Autodesk Inventor part; units mm, degrees
ref_plane "YZ Plane" through (0, 0, 0) normal (1, 0, 0) x (0, 1, 0)
ref_plane "XZ Plane" through (0, 0, 0) normal (0, 1, 0) x (-1, 0, 0)
ref_plane "XY Plane" through (0, 0, 0) normal (0, 0, 1) x (1, 0, 0)
sketch "스케치1" plane through (0, 0, 0) normal (0, 0, 1) x (1, 0, 0)
  circle A0 centre (88.547, 17.9758) radius 1.2
  circle A1 centre (86.2038, 23.6326) radius 1.2
  circle A2 centre (80.547, 25.9758) radius 1.2
  circle A3 centre (74.8901, 23.6326) radius 1.2
  circle A4 centre (72.547, 17.9758) radius 1.2
  circle A5 centre (80.547, 17.9758) radius 5.8
  arc A6 (69.647, 17.9758) -> (74.747, 17.9758) centre (72.197, 18.4832) ccw
  arc A7 (86.347, 17.9758) -> (91.447, 17.9758) centre (88.897, 18.4832) ccw
  line L0 (69.647, 17.9758) -> (91.447, 17.9758)
  line L1 (91.447, 17.9758) -> (91.447, 37.9758)
  line L2 (91.447, 37.9758) -> (69.647, 37.9758)
  line L3 (69.647, 37.9758) -> (69.647, 17.9758)
  line L4 (69.647, 37.9758) -> (99.4042, 37.9758) construction
  line L5 (69.647, 37.9758) -> (91.447, 37.9758)
  line L6 (91.447, 37.9758) -> (91.447, 52.9758)
  line L7 (91.447, 52.9758) -> (69.647, 52.9758)
  line L8 (69.647, 52.9758) -> (69.647, 37.9758)
  line L9 (69.647, 52.9758) -> (69.647, 52.9758)
  line L10 (91.447, 52.9758) -> (91.447, 52.9758)
  circle A8 centre (69.647, 52.9758) radius 21.8
  line L11 (69.647, 52.9758) -> (54.232, 68.3907)
  point P0 (0, 0)
  point P1 (80.547, 17.9758)
  point P2 (80.547, 17.9758)
  point P3 (69.647, 57.9758)
  point P4 (85.4659, 37.9758)
  point P5 (69.647, 31.1758)
  dimension "d4" = 2.6
  dimension "d5" = 2.6
  dimension "d6" = 20
  dimension "d9" = 15
  dimension "d19" = 0
  dimension "d20" = 0
  dimension "d30" = 135
extrude "돌출1" add sketch "스케치1" along normal blind 6 contours L0 A7 A0 | A0 L0 A5 A4 L3 A8 L2 L1 | L2 A8 L6 | A6 L0 A4 | A8 L3 L2 | L2 L8 L7 A8 | L7 L11 A8
sketch "스케치2" plane through (0, 0, 6) normal (0, 0, 1) x (1, 0, 0)
  arc A0 (69.647, 17.9758) -> (74.747, 17.9758) centre (72.197, 18.4832) ccw
  arc A1 (86.347, 17.9758) -> (74.747, 17.9758) centre (80.547, 17.9758) ccw
  arc A2 (86.347, 17.9758) -> (91.447, 17.9758) centre (88.897, 18.4832) ccw
  circle A3 centre (88.547, 17.9758) radius 1.2
  circle A4 centre (72.547, 17.9758) radius 1.2
  circle A5 centre (80.547, 25.9758) radius 1.2
  circle A6 centre (86.2038, 23.6326) radius 1.2
  circle A7 centre (74.8901, 23.6326) radius 1.2
  circle A8 centre (72.547, 17.9758) radius 1.35
  circle A9 centre (74.8901, 23.6326) radius 1.35
  circle A10 centre (80.547, 25.9758) radius 1.35
  circle A11 centre (86.2038, 23.6326) radius 1.35
  circle A12 centre (88.547, 17.9758) radius 1.35
  arc A13 (91.447, 52.9758) -> (54.232, 68.3907) centre (69.647, 52.9758) ccw
  line L0 (69.647, 52.9758) -> (69.647, 17.9758)
  line L1 (91.447, 17.9758) -> (91.447, 52.9758)
  line L2 (54.232, 68.3907) -> (69.647, 52.9758)
  point P0 (0, 0)
  dimension "d12" = 2.7
  dimension "d13" = 2.7
  dimension "d14" = 2.7
  dimension "d15" = 2.7
  dimension "d16" = 2.7
extrude "돌출2" cut sketch "스케치2" against normal blind 6 contours A3 | A4 | A5 | A6 | A7 | A8 | A9 | A10 | A11 | A12
fillet "모깎기1" radius 1 1 edges at (54.232, 68.3907, 3)
sketch "스케치3" plane through (0, 0, 6) normal (0, 0, 1) x (1, 0, 0)
  arc A0 (54.991, 69.114) -> (54.9562, 67.6666) centre (55.6633, 68.3737) ccw
  line L0 (54.9562, 67.6666) -> (69.647, 52.9758)
  line L1 (69.647, 52.9758) -> (69.647, 17.9758)
  arc A1 (69.647, 17.9758) -> (74.747, 17.9758) centre (72.197, 18.4832) ccw
  arc A2 (86.347, 17.9758) -> (74.747, 17.9758) centre (80.547, 17.9758) ccw
  arc A3 (86.347, 17.9758) -> (91.447, 17.9758) centre (88.897, 18.4832) ccw
  line L2 (91.447, 17.9758) -> (91.447, 52.9758)
  arc A4 (91.447, 52.9758) -> (54.991, 69.114) centre (69.647, 52.9758) ccw
  circle A5 centre (86.2038, 23.6326) radius 1.35
  circle A6 centre (88.547, 17.9758) radius 1.35
  circle A7 centre (80.547, 25.9758) radius 1.35
  circle A8 centre (72.547, 17.9758) radius 1.35
  circle A9 centre (74.8901, 23.6326) radius 1.35
  line L3 (85.547, 49.9758) -> (75.547, 49.9758)
  line L4 (75.547, 49.9758) -> (75.547, 55.9758)
  line L5 (75.547, 55.9758) -> (85.547, 55.9758)
  line L6 (85.547, 55.9758) -> (85.547, 49.9758)
  line L7 (85.547, 49.9758) -> (75.547, 55.9758) construction
  line L8 (75.547, 49.9758) -> (85.547, 55.9758) construction
  point P0 (0, 0)
  point P1 (80.547, 52.9758)
  dimension "d22" = 10
  dimension "d23" = 6
extrude "돌출3" cut sketch "스케치3" against normal blind 6 contours L3 L4 L5 L6
sketch "스케치4" plane through (0, 0, 6) normal (0, 0, 1) x (1, 0, 0)
  line L0 (75.547, 49.9758) -> (75.547, 55.9758)
  line L1 (75.547, 55.9758) -> (85.547, 55.9758)
  line L2 (85.547, 55.9758) -> (85.547, 49.9758)
  line L3 (85.547, 49.9758) -> (75.547, 49.9758)
  arc A0 (54.991, 69.114) -> (54.9562, 67.6666) centre (55.6633, 68.3737) ccw
  line L4 (54.9562, 67.6666) -> (69.647, 52.9758)
  line L5 (69.647, 52.9758) -> (69.647, 17.9758)
  arc A1 (69.647, 17.9758) -> (74.747, 17.9758) centre (72.197, 18.4832) ccw
  arc A2 (86.347, 17.9758) -> (74.747, 17.9758) centre (80.547, 17.9758) ccw
  arc A3 (86.347, 17.9758) -> (91.447, 17.9758) centre (88.897, 18.4832) ccw
  line L6 (91.447, 17.9758) -> (91.447, 52.9758)
  arc A4 (91.447, 52.9758) -> (54.991, 69.114) centre (69.647, 52.9758) ccw
  circle A5 centre (86.2038, 23.6326) radius 1.35
  circle A6 centre (88.547, 17.9758) radius 1.35
  circle A7 centre (80.547, 25.9758) radius 1.35
  circle A8 centre (72.547, 17.9758) radius 1.35
  circle A9 centre (74.8901, 23.6326) radius 1.35
  circle A10 centre (72.547, 52.9758) radius 1.35
  circle A11 centre (88.547, 52.9758) radius 1.35
  point P0 (0, 0)
  point P1 (75.547, 52.9758)
  dimension "d26" = 2.7
  dimension "d27" = 2.7
  dimension "d31" = 3
extrude "돌출4" cut sketch "스케치4" against normal blind 6 contours A10 | A11
sketch "스케치5" plane through (0, 0, 6) normal (0, 0, 1) x (1, 0, 0)
  line L0 (75.547, 55.9758) -> (75.547, 49.9758)
  circle A0 centre (75.547, 55.9758) radius 0.75
  circle A1 centre (85.3736, 55.9758) radius 0.75
  line L1 (75.547, 49.9758) -> (85.547, 49.9758)
  circle A2 centre (75.547, 49.9758) radius 0.75
  line L2 (85.547, 49.9758) -> (85.547, 55.9758)
  circle A3 centre (85.547, 49.9758) radius 0.75
  point P0 (0, 0)
  point P1 (85.547, 50.7258)
  point P2 (84.797, 49.9758)
  dimension "d32" = 1.5
  dimension "d33" = 1.5
  dimension "d34" = 1.5
  dimension "d35" = 1.5
extrude "돌출5" cut sketch "스케치5" against normal blind 10 contours A1 | L1 L2 A3 | A2 L1 L0 | L0 L1 A2 | A0 picked at (85.0543, 49.916)
properties part number "frame_hand1" material "PMMA 플라스틱"
Can you work these out from the model? Positions are in its coordinate system, mm. A direction names the side the tool comes from. Round coordinates to 2 decimals unless told otherwise and drop trailing zeros. Write each loop counter-clockwise with the first axis right and the second up, starting at its lowest first coordinate (ties: lowest second). Pieces come first, ordered by that corner, then holes. Notation, with made-up numbers: M -3.75,7 L 53.25,7 A32 cw 53.25,45 Z; hole C 67,-5.75 d9. An arc over 180 degrees is marked long. Use a Markdown table: item, result.
Item 1: For pin 1 Ø1.5 at (x, z) = (59, 3.5) entering from -Y; pin 2 Ø1.5 at (x, z) = (84, 1.5) entering from -Y; pin 3 Ø1 at (y, z) = (55, 3) entering from +X, each with a flat end and sliding along its axis, tell me the tip position at first contact or that it passes through.
Found:
| item | result |
|---|---|
| pin 1 | stops at y = 62.87 |
| pin 2 | stops at y = 21.97 |
| pin 3 | stops at x = 91.39 |
Item 2: Which directions (+Z, -Z, +X, -X, +Y, -Y) give clear straight access to the entire face, cutting with the end or side of a thin tool? Please do faces 4 (the face through (77, 46, 0)), 5 (the face through (80, 55.976, 3)).
Found:
| item | result |
|---|---|
| face 4 | -Z, +X, -X, +Y, -Y |
| face 5 | +Z, -Z |
Item 3: I want a section at D-D (x = 77.5). List the corners of the cut face in (y, z) for me.
Found:
| item | result |
|---|---|
| outline | M 22.91,0 L 49.98,0 L 49.98,6 L 22.91,6 Z; M 55.98,0 L 73.31,0 L 73.31,6 L 55.98,6 Z |
Item 4: I want a section at A-A (x = 83). List the corners of the cut face in (y, z) for me.
Found:
| item | result |
|---|---|
| outline | M 23.23,0 L 49.98,0 L 49.98,6 L 23.23,6 Z; M 55.98,0 L 70.21,0 L 70.21,6 L 55.98,6 Z |
Item 5: I want a section at C-C (y = 32). List the corners of the cut face in (x, z) for me.
Found:
| item | result |
|---|---|
| outline | M 69.65,0 L 91.45,0 L 91.45,6 L 69.65,6 Z |
Item 6: If I drill on line 1 along X through (y, z) = (52, 5.55); line 2 along Y through (x, z) = (80, 4.25); line 3 along X through (y, z) = (45.5, 2.8), over which ranges is the centre line in solid material (lowest first)? Write a range as [from, to].
Found:
| item | result |
|---|---|
| line 1 | x = [69.65, 71.61], [73.48, 75.55], [85.55, 87.61], [89.48, 91.45] |
| line 2 | y = [23.75, 24.74], [27.21, 49.98], [55.98, 72.16] |
| line 3 | x = [69.65, 91.45] |
Item 7: I want a section at B-B (z = 1.35). State how many separate pieces and enclosed holes the cut face has, and give its area (3 significant figures).
Found:
| item | result |
|---|---|
| separate pieces | 1 |
| enclosed holes | 8 |
| area | 1,180 mm2 |
Item 8: We'd pull the mould along X, two halves only. Please class faces 1 (the face through (78.15, 73.05, 2.96)), 2 (the face through (54.664, 68.409, 3.042)), 3 (the face through (81, 49.976, 3)): released by +X, released by -X, zero draft, split by the parting line, or undercut.
Found:
| item | result |
|---|---|
| face 1 | split by the parting line |
| face 2 | released by -X |
| face 3 | undercut |
